Read the model definition and answer for the solid it produces. Units are mm, in the model's axes. Face numbers are marked on the shaded views. Give positions to 0.01 mm unless a question says otherwise; leave off trailing zeros. Write each loop counter-clockwise with the first axis right and the second up, starting at its lowest first coordinate (ties: lowest second). Pieces come first, ordered by that corner, then holes. Notation, with made-up numbers: M -22.5,77 L 12.5,77 A17 cw 12.5,83 Z; hole C 42.25,89.5 d4. An arc over 180 degrees is marked long. Put each result on its own line as item: value.
from build123d import *

# Parameters (mm, degrees)
F0_R     = 3.25
F0_R_2   = 5.25
F0_R_3   = 2.75
F1_DEPTH = 4
F2_R     = 6
F3_R     = 4


with BuildPart() as f1:
    # F0 (on Top) → F1 (new body)
    with BuildSketch(Plane.XY):
        with BuildLine():
            Line((-35.216862, 4.573831), (-4.908502, -10.122703))
            ThreePointArc((-4.908502, -10.122703), (9.185091, -6.495891), (7.908829, 8.000807))
            Line((7.908829, 8.000807), (-22.747156, 38.304369))
            Line((-22.747156, 38.304369), (-35.216862, 44.119088))
            Line((-35.216862, 44.119088), (-35.216862, 4.573831))
        make_face()
        with Locations((-29.466862, 14.856111)):
            Circle(F0_R, mode=Mode.SUBTRACT)
        Circle(F0_R_2, mode=Mode.SUBTRACT)
        with Locations((-26.216862, 34.08337)):
            Circle(F0_R_3, mode=Mode.SUBTRACT)
    extrude(amount=F1_DEPTH)

    # F2
    f2_edges = [f1.edges().sort_by_distance(p)[0] for p in [
        (-22.747156, 38.304369, 2),
        (-35.216862, 4.573831, 2),
    ]]
    fillet(f2_edges, radius=F2_R)

    # F3
    f3_edges = [f1.edges().sort_by_distance(p)[0] for p in [
        (-35.216862, 44.119088, 2),
    ]]
    fillet(f3_edges, radius=F3_R)


solid = f1.part
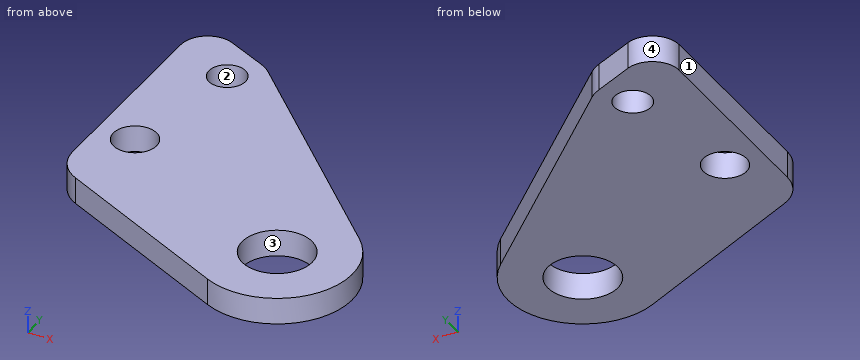
(1) Section B-B on z = 2.4 is taken. Determine the outline of the cut face in (x, y).
Result:
outline: M -35.22,8.33 A6 ccw -31.83,2.93 L -4.91,-10.12 A11.25 ccw 7.91,8 L -22.01,37.57 A6 ccw -23.69,38.74 L -29.53,41.47 A4 ccw -35.22,37.84 Z; hole C -29.47,14.86 d6.5; hole C -26.22,34.08 d5.5; hole C 0,0 d10.5
(2) Straight lines are drawn through the part: line 1 along Y through (x, z) = (-27, 1.9); line 2 along Y through (x, z) = (-29.5, 3.8); line 3 along Y through (x, z) = (-4, 0.5). For each, find the intervals that lie inside material, in ascending order. Write a range as from..to.
Result:
line 1: y = 0.59..12.74, 16.97..31.45, 36.72..40.29
line 2: y = 1.8..11.61, 18.11..41.45
line 3: y = -10.51..-3.4, 3.4..19.77
(3) Section C-C on x = 0 is taken. Determine the outline of the cut face in (y, z), and give its area (3 significant figures).
Result:
outline: M -11.25,0 L -5.25,0 L -5.25,4 L -11.25,4 Z; M 5.25,0 L 15.82,0 L 15.82,4 L 5.25,4 Z
area: 66.3 mm²
(4) Section A-A on y = -3 is taken. Determine the outline of the cut face in (x, z), and give its area (3 significant figures).
Result:
outline: M -19.6,0 L -4.31,0 L -4.31,4 L -19.6,4 Z; M 4.31,0 L 10.84,0 L 10.84,4 L 4.31,4 Z
area: 87.3 mm²
(5) For a pull along Y with two mould halves and no side action, classify the marked faces 1, 2, 3 and 4 as +Y half, -Y half, draft (parallel to the pull), parting line (faces both ways), or undercut.
Result:
face 1: draft
face 2: undercut
face 3: undercut
face 4: +Y half
(6) Section D-D on x = -6 is taken. Determine the outline of the cut face in (y, z).
Result:
outline: M -9.59,0 L 21.75,0 L 21.75,4 L -9.59,4 Z
(7) Given pin 1 Ø8.5 at (x, y) = (0, 0) entering from -Z, flat-ended and moving along its own axis, determine where the tip first touches the part or whether it passes through.
Result:
pin 1: passes through
